Read the model definition and answer for the solid it produces. Units are mm, in the model's axes. Face numbers are marked on the shaded views. Give positions to 0.01 mm unless a question says otherwise; leave off trailing zeros. Write each loop counter-clockwise with the first axis right and the second up, starting at its lowest first coordinate (ties: lowest second). Pieces come first, ordered by that corner, then holes. Notation, with made-up numbers: (-6, 1) -> (37, 1) arc R19 cw to (37, 10) -> close; hole circle Ø4 at (-8, 82.25). An arc over 180 degrees is marked (long way). Write item = value, one per line.
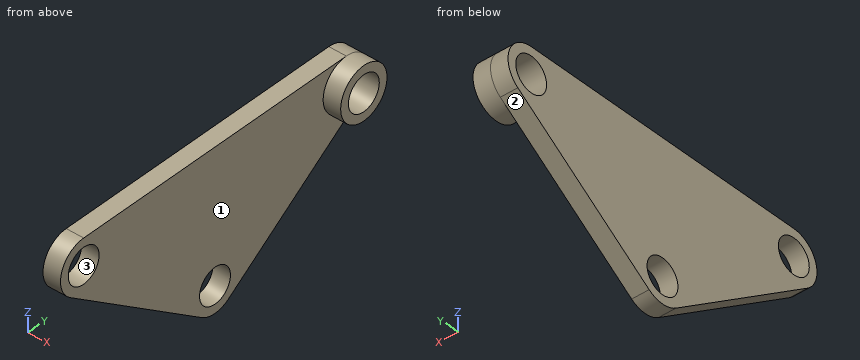
from build123d import *

# Parameters (mm, degrees)
EXTRUDE_1_DEPTH          = 2
EXTRUDE_START            = 2
SKETCH_1_4_R             = 3
EXTRUDE_2_DEPTH          = 2
CUT_EXTRUDE_1_DEPTH      = 45.045431091
CUT_EXTRUDE_1_DEPTH_BACK = 45.045431091
SKETCH_1_3_R             = 2


with BuildPart() as part:
    # 草图1 → 凸台-拉伸1 (new body)
    with BuildSketch(Plane(origin=(0, 0, 0), x_dir=(0, 0, -1), z_dir=(1, 0, 0))):
        with BuildLine():
            Line((17.45090359, -18.269950407), (5.45090359, -1.269950407))
            ThreePointArc((5.45090359, -1.269950407), (2.092451315, -0.140567297), (0, -3))
            Line((0, -3), (0, -37))
            ThreePointArc((0, -37), (2.092451315, -39.859432703), (5.45090359, -38.730049593))
            Line((5.45090359, -38.730049593), (17.45090359, -21.730049593))
            ThreePointArc((17.45090359, -21.730049593), (18, -20), (17.45090359, -18.269950407))
        make_face()
    extrude(amount=EXTRUDE_1_DEPTH)

    # 草图1<4> → 凸台-拉伸2 (add)
    with BuildSketch(Plane(origin=(0, 0, 0), x_dir=(0, 0, -1), z_dir=(1, 0, 0)).offset(EXTRUDE_START)):
        with Locations(Location((3, -3, 0), (0, 0, 180))):
            Circle(SKETCH_1_4_R)
    extrude(amount=EXTRUDE_2_DEPTH)

    # 草图1<3> → 切除-拉伸1 (cut, two sides: drawn at the far end of the back side and taken through both)
    with BuildSketch(Plane(origin=(0, 0, 0), x_dir=(0, 0, -1), z_dir=(1, 0, 0)).offset(-CUT_EXTRUDE_1_DEPTH_BACK)):
        with Locations((3, -3)):
            Circle(SKETCH_1_3_R)
        with Locations((15, -20)):
            Circle(SKETCH_1_3_R)
        with Locations((3, -37)):
            Circle(SKETCH_1_3_R)
    extrude(amount=CUT_EXTRUDE_1_DEPTH + CUT_EXTRUDE_1_DEPTH_BACK, mode=Mode.SUBTRACT)


solid = part.part
(1) The part is cut by section A-A on z = -3. Determine the outline of the cut face in (x, y).
Checks:
outline = (0, -40) -> (2, -40) -> (2, -39) -> (0, -39) -> close; (0, -35) -> (2, -35) -> (2, -6) -> (4, -6) -> (4, -5) -> (0, -5) -> close; (0, -1) -> (4, -1) -> (4, 0) -> (0, 0) -> close
(2) Consider L1, parallel to Z at x = 2.4, y = -3; L2, parallel to Y at x = 1.15, z = -3.5. Determine where each line is inside the solid, lowest interval first.
Checks:
L1 = -6 to -5, -1 to 0
L2 = -39.96 to -38.94, -35.06 to -4.94, -1.06 to -0.04
(3) The part is cut by section B-B on y = -20. Determine the outline of the cut face in (x, z).
Checks:
outline = (0, -18) -> (2, -18) -> (2, -17) -> (0, -17) -> close; (0, -13) -> (2, -13) -> (2, 0) -> (0, 0) -> close
(4) For a pull along Y with two mould halves and no side action, classify the marked faces 1, 2 and 3 as released by +Y, released by -Y, zero draft, split by the parting line, or undercut.
Checks:
face_1 = zero draft
face_2 = released by +Y
face_3 = undercut
(5) Given P1, Ø5, axis at y = -37, z = -3, coming from the +X side, flat-ended and moving along its own axis, determine where the tip first touches the part or whether it passes through.
Checks:
P1 = 2
(6) The part is cut by section C-C on x = 1.3. Determine the outline of the cut face in (y, z).
Checks:
outline = (-38.73, -5.45) -> (-21.73, -17.45) arc R3 ccw to (-18.27, -17.45) -> (-1.27, -5.45) arc R3 ccw to (-3, 0) -> (-37, 0) arc R3 ccw to start; hole circle Ø4 at (-37, -3); hole circle Ø4 at (-20, -15); hole circle Ø4 at (-3, -3)
(7) The part is cut by section D-D on x = 3.05. Determine the outline of the cut face in (y, z).
Checks:
outline = circle Ø6 at (-3, -3); hole circle Ø4 at (-3, -3)
